from build123d import *

# Parameters (mm, degrees)
SALIENTE_EXTRUIR1_DEPTH = 140
CROQUIS2_R              = 4.029640203
CORTAR_EXTRUIR1_DEPTH   = 140


with BuildPart() as part:
    # Croquis1 → Saliente-Extruir1 (new body)
    with BuildSketch(Plane.XY):
        Polygon((-1, -25.4), (-2.773222037, -25.4), (-6.35, -10.576393443), (-6.35, 25.4), (6.35, 25.4), (6.35, -10.576393443), (2.773222037, -25.4), (1, -25.4), (1, -19.4), (-1, -19.4), align=None)
    extrude(amount=SALIENTE_EXTRUIR1_DEPTH)

    # Croquis2 → Cortar-Extruir1 (cut)
    with BuildSketch(Plane(origin=(6.35, 0, 0), x_dir=(0, 0, -1), z_dir=(1, 0, 0))):
        with Locations((-70, 15.4)):
            Circle(CROQUIS2_R)
    extrude(amount=-CORTAR_EXTRUIR1_DEPTH, mode=Mode.SUBTRACT)


solid = part.part
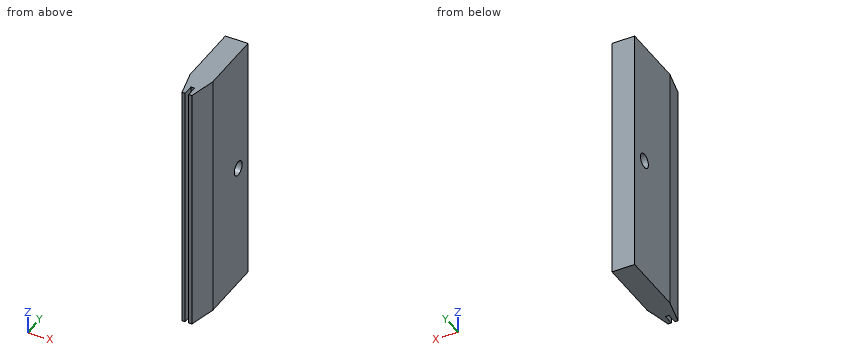
The listing builds one solid part. Answer for the finished solid, in the listing's coordinates (mm). Round coordinates to 2 decimals unless told otherwise and drop trailing zeros. Loops run counter-clockwise (first coordinate to the right, second up) from the corner with the lowest first, then second, coordinate; pieces in that order, holes last. Notation, with made-up numbers: M 28.25,36.25 L 41.25,36.25 A13 ccw 41.25,52.25 Z; hole C 54,81 d10. An arc over 180 degrees is marked long. Return JSON: item names as keys, results as strings.
Q1. Find section C-C, the plane x = -4. Determine the outline of the cut face in (y, z).
Results list:
{"outline": "M -20.32,0 L 25.4,0 L 25.4,140 L -20.32,140 Z; hole C 15.4,70 d8.06"}
Q2. Find section D-D, the plane y = -13.5. Determine the outline of the cut face in (x, z).
Results list:
{"outline": "M -5.64,0 L 5.64,0 L 5.64,140 L -5.64,140 Z"}
Q3. Find section A-A, the plane y = 15.4. Determine the outline of the cut face in (x, z).
Results list:
{"outline": "M -6.35,0 L 6.35,0 L 6.35,65.97 L -6.35,65.97 Z; M -6.35,74.03 L 6.35,74.03 L 6.35,140 L -6.35,140 Z"}
Q4. Find the intervals of material crossed by line 1 along Y through (x, z) = (-1.5, 70); line 2 along Y through (x, z) = (0.75, 70); line 3 along Y through (x, z) = (0.75, 97), in increasing order. Write a range as from..to.
Results list:
{"line 1": "y = -25.4..11.37, 19.43..25.4", "line 2": "y = -19.4..11.37, 19.43..25.4", "line 3": "y = -19.4..25.4"}
Q5. Find section B-B, the plane z = 70. Determine the outline of the cut face in (x, y).
Results list:
{"outline": "M -6.35,-10.58 L -2.77,-25.4 L -1,-25.4 L -1,-19.4 L 1,-19.4 L 1,-25.4 L 2.77,-25.4 L 6.35,-10.58 L 6.35,11.37 L -6.35,11.37 Z; M -6.35,19.43 L 6.35,19.43 L 6.35,25.4 L -6.35,25.4 Z"}
Q6. Each of these flat-tipped pins is pushed along its axis until it touches: pin 1 Ø6.5 at (y, z) = (-22.5, 67) entering from +X; pin 2 Ø1 at (x, z) = (0, 55) entering from -Y; pin 3 Ø6.5 at (y, z) = (-24, 78) entering from -X. Where does it stop, or does it pass through?
Results list:
{"pin 1": "stops at x = 4.26", "pin 2": "stops at y = -19.4", "pin 3": "stops at x = -3.9"}
